```python
from build123d import *

# Parameters (mm, degrees)
PAD_DEPTH     = 15
SKETCH002_R   = 1.6
SKETCH002_R_2 = 2
POCKET_DEPTH  = 27.201
CHAMFER_SIZE  = 2


with BuildPart() as bodyinner:
    # Sketch001 → Revolution (revolve)
    with BuildSketch(Plane.XY):
        Polygon((0, 0), (8, 0), (8, 9), (2.4, 9), (2.4, 35), (0, 35), align=None)
    revolve(axis=Axis((0, 0, 0), (0, 1, 0)))


with BuildPart() as chamfer_body:
    # Sketch → Pad (new body, symmetric)
    with BuildSketch(Plane.XY):
        Polygon((-15, 17.1), (15, 17.1), (15, 7), (35.2, 7), (35.2, 27.2), (42.2, 27.2), (42.2, 0), (-15, 0), align=None)
    extrude(amount=PAD_DEPTH, both=True)

    # Sketch002 → Pocket (cut, through all)
    with BuildSketch(Plane.XZ):
        with Locations((-9, 9)):
            Circle(SKETCH002_R)
        with Locations((9, 9)):
            Circle(SKETCH002_R)
        with Locations((9, -9)):
            Circle(SKETCH002_R)
        with Locations((-9, -9)):
            Circle(SKETCH002_R)
        with Locations((25.1, 0)):
            Circle(SKETCH002_R_2)
    extrude(amount=-POCKET_DEPTH, mode=Mode.SUBTRACT)

    # Cut: cut BodyInner
    add(bodyinner.part, mode=Mode.SUBTRACT)

    # Chamfer
    chamfer_edges = [chamfer_body.edges().sort_by_distance(p)[0] for p in [
        (-15, 17.1, 0),
        (-15, 0, 0),
        (42.2, 0, 0),
        (42.2, 27.2, 0),
    ]]
    chamfer(chamfer_edges, length=CHAMFER_SIZE)


solid = chamfer_body.part
```
Design review of the part built by this model. Coordinates are the model's own, in mm. A direction names the side the tool comes from. Coordinates: 2 decimals unless noted, no trailing zeros. Write each loop counter-clockwise with the first axis right and the second up, starting at its lowest first coordinate (ties: lowest second). Pieces come first, ordered by that corner, then holes. Notation, with made-up numbers: M 52,69 L 92,69 A20 ccw 92,100 Z; hole C 89,86 d10. An arc over 180 degrees is marked long. Answer as a JSON object with one key per item and string values.
Item 1: Draft analysis for pull direction Z (two halves, no side actions). For faces 1 (the flat face through (35.2, 17, 0)), 2 (the cylindrical face through (-1.73, 4.56, 7.81)), 3 (the flat face through (14, 11, 15)), state which applies: pulls with the +Z half, pulls with the -Z half, needs draft (parallel to the pull), parting line crosses it, or undercut.
Outcome:
{"face 1": "needs draft", "face 2": "undercut", "face 3": "pulls with the +Z half"}
Item 2: Insertion check: pin 1 Ø3 at (x, z) = (0.5, 2) entering from +Y; pin 2 Ø2.5 at (x, z) = (-9, 9) entering from -Y; pin 3 Ø13 at (x, z) = (0, 0) entering from -Y; pin 4 Ø5 at (x, z) = (21, 1.5) entering from +Y. Each pin has a flat end and moves straight along its axis. Give the tip position at first contact, or say it passes through.
Outcome:
{"pin 1": "y = 17.1", "pin 2": "through", "pin 3": "y = 9", "pin 4": "y = 7"}
Item 3: Add section A-A, the plane x = -9. Give the boundary of the cut face in (y, z).
Outcome:
{"outline": "M 0,-15 L 17.1,-15 L 17.1,-10.6 L 0,-10.6 Z; M 0,-7.4 L 17.1,-7.4 L 17.1,7.4 L 0,7.4 Z; M 0,10.6 L 17.1,10.6 L 17.1,15 L 0,15 Z"}
Item 4: Wall thickness on probe 1 along Z at (x, y) = (-9, 11.5); probe 2 along Z at (x, y) = (25, 5); probe 3 along Z at (x, y) = (0, 13.5): over which ranges is each line inside the solid? List them lowest first.
Outcome:
{"probe 1": "-15 to -10.6, -7.4 to 7.4, 10.6 to 15", "probe 2": "-15 to -2, 2 to 15", "probe 3": "-15 to -2.4, 2.4 to 15"}
Item 5: Machinability: for faces 4 (the flat face through (4, 17.1, 0)), 5 (the flat face through (-2, 9, 2)), 6 (the flat face through (41.2, 1, -0.2)), which of the approach directions +Z, -Z, +X, -X, +Y, -Y give a long, thin tool a straight path to every point of the face, cutting with its end or side? Answer none if there is none.
Outcome:
{"face 4": "+Z, -Z, -X, +Y", "face 5": "-Y", "face 6": "+Z, -Z, +X, -Y"}
Item 6: Add section B-B, the plane z = 9. Give the boundary of the cut face in (x, y).
Outcome:
{"outline": "M -15,2 L -13,0 L -10.6,0 L -10.6,17.1 L -13,17.1 L -15,15.1 Z; M -7.4,0 L 7.4,0 L 7.4,17.1 L -7.4,17.1 Z; M 10.6,0 L 40.2,0 L 42.2,2 L 42.2,25.2 L 40.2,27.2 L 35.2,27.2 L 35.2,7 L 15,7 L 15,17.1 L 10.6,17.1 Z"}
Item 7: Add section D-D, the plane y = 23. Give the boundary of the cut face in (x, z), and give its area (3 significant figures).
Outcome:
{"outline": "M 35.2,-15 L 42.2,-15 L 42.2,15 L 35.2,15 Z", "area": "210 mm²"}
Item 8: Add section C-C, the plane x = 0. Give the boundary of the cut face in (y, z), and give its area (3 significant figures).
Outcome:
{"outline": "M 0,-15 L 17.1,-15 L 17.1,-2.4 L 9,-2.4 L 9,-8 L 0,-8 Z; M 0,8 L 9,8 L 9,2.4 L 17.1,2.4 L 17.1,15 L 0,15 Z", "area": "330 mm²"}
